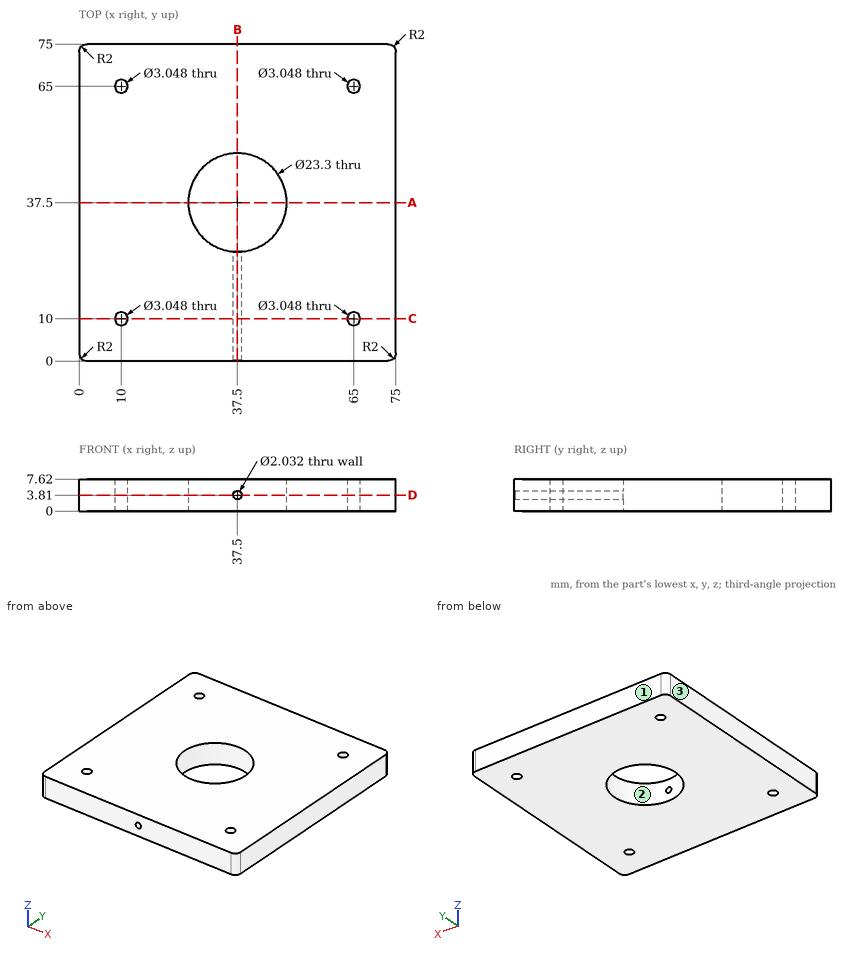
Verification items for this drawing (mm, ordinates from the low corner). Give positions to 0.01 mm unless a question says otherwise; leave off trailing zeros. Loops run counter-clockwise (first coordinate to the right, second up) from the corner with the lowest first, then second, coordinate; pieces in that order, holes last. Notation, with made-up numbers: M -21.5,-36.5 L -17.5,-36.5 A12 ccw -17.5,-23.5 Z; hole C 66,39.5 d2. An arc over 180 degrees is marked long. Write item = value, one per line.
(1) Sectioned sample at C-C, the plane y = 10. Record the cut outline in (x, z).
Answer below:
outline = M 0,0 L 8.48,0 L 8.48,7.62 L 0,7.62 Z; M 11.52,0 L 63.48,0 L 63.48,7.62 L 11.52,7.62 Z; M 66.52,0 L 75,0 L 75,7.62 L 66.52,7.62 Z; hole C 37.5,3.81 d2.03
(2) Sectioned sample at D-D, the plane z = 3.81. Record the cut outline in (x, y), plus the area to 3 significant figures.
Answer below:
outline = M 0,2 A2 ccw 2,0 L 36.48,0 L 36.48,25.89 A11.65 cw long 38.52,25.89 L 38.52,0 L 73,0 A2 ccw 75,2 L 75,73 A2 ccw 73,75 L 2,75 A2 ccw 0,73 Z; hole C 10,10 d3.05; hole C 10,65 d3.05; hole C 65,10 d3.05; hole C 65,65 d3.05
area = 5,110 mm2
(3) Material ranges on line 1 (Y direction, x = 10, z = 0.5); line 2 (Y direction, x = 11, z = 4); line 3 (Y direction, x = 33, z = 3.5), recorded low to high. Write a range as [from, to].
Answer below:
line_1 = [0, 8.48], [11.52, 63.48], [66.52, 75]
line_2 = [0, 8.85], [11.15, 63.85], [66.15, 75]
line_3 = [0, 26.75], [48.25, 75]
(4) Release check for a two-part mould opening along Y. For the marked faces 1, 2 and 3 record: released by +Y, released by -Y, zero draft, split by the parting line, or undercut.
Answer below:
face_1 = released by +Y
face_2 = undercut
face_3 = zero draft
(5) Sectioned sample at B-B, the plane x = 37.5. Record the cut outline in (y, z).
Answer below:
outline = M 0,0 L 25.85,0 L 25.85,2.79 L 0,2.79 Z; M 0,4.83 L 25.85,4.83 L 25.85,7.62 L 0,7.62 Z; M 49.15,0 L 75,0 L 75,7.62 L 49.15,7.62 Z
(6) Sectioned sample at A-A, the plane y = 37.5. Record the cut outline in (x, z), plus the area to 3 significant figures.
Answer below:
outline = M 0,0 L 25.85,0 L 25.85,7.62 L 0,7.62 Z; M 49.15,0 L 75,0 L 75,7.62 L 49.15,7.62 Z
area = 394 mm2
